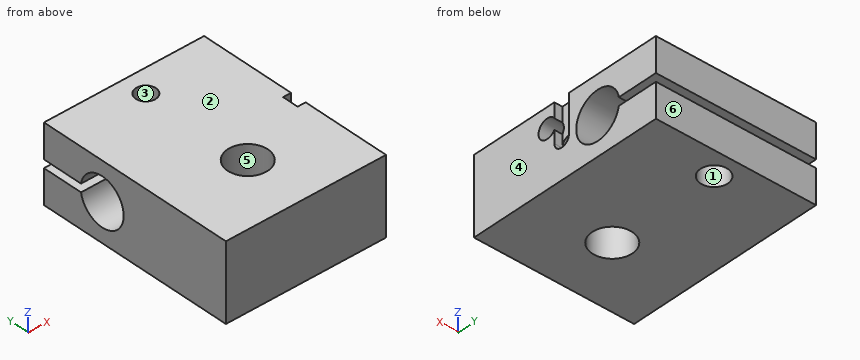
```python
from build123d import *

# Parameters (mm, degrees)
F0_W     = 20
F0_H     = 25
F0_R     = 2.5
F0_R_2   = 1.25
F1_DEPTH = 4.75
F3_DEPTH = 20.001
F4_R     = 1.7
F5_DEPTH = 4.25
F6_R     = 1
F6_R_2   = 1.190625
F7_DEPTH = 7
F8_W     = 2
F8_H     = 4.7499998814
F9_DEPTH = 1


with BuildPart() as f1:
    # F0 (on Top) → F1 (new body, symmetric)
    with BuildSketch(Plane.XY):
        Rectangle(F0_W, F0_H)
        with Locations((0, -4.5)):
            Circle(F0_R, mode=Mode.SUBTRACT)
        with Locations((0, 9.5)):
            Circle(F0_R_2, mode=Mode.SUBTRACT)
    extrude(amount=F1_DEPTH, both=True)

    # F2 (on face) → F3 (cut, through all)
    with BuildSketch(Plane.YZ.offset(10)):
        with BuildLine():
            ThreePointArc((7.407318352, -0.5), (7.43931022, -0.2509092082), (7.45, 0))
            ThreePointArc((7.45, 0), (7.43931022, 0.2509092082), (7.407318352, 0.5))
            Line((7.407318352, 0.5), (7.407318352, -0.5))
        make_face()
        with BuildLine():
            ThreePointArc((7.407318352, 0.5), (7.43931022, 0.2509092082), (7.45, 0))
            ThreePointArc((7.45, 0), (7.43931022, -0.2509092082), (7.407318352, -0.5))
            Line((7.407318352, -0.5), (12.5, -0.5))
            Line((12.5, -0.5), (12.5, 0.5))
            Line((12.5, 0.5), (7.407318352, 0.5))
        make_face()
        with BuildLine():
            Line((7.407318352, -0.5), (7.407318352, 0.5))
            ThreePointArc((7.407318352, 0.5), (1.55, 0), (7.407318352, -0.5))
        make_face()
    extrude(amount=-F3_DEPTH, mode=Mode.SUBTRACT)

    # F4 (on face) → F5 (cut, through all)
    with BuildSketch(Plane(origin=(0, 0, -4.75), x_dir=(1, 0, 0), z_dir=(0, 0, -1))):
        with Locations((0, -9.5)):
            Circle(F4_R)
    extrude(amount=-F5_DEPTH, mode=Mode.SUBTRACT)

    # F6 (on face) → F7 (cut)
    with BuildSketch(Plane.YZ.offset(10)):
        with Locations((-0.45, 0)):
            Circle(F6_R)
        with Locations((-2.4343134833, 2.25)):
            Circle(F6_R_2)
    extrude(amount=-F7_DEPTH, mode=Mode.SUBTRACT)

    # F8 (on face) → F9 (cut)
    with BuildSketch(Plane.YZ.offset(10)):
        with Locations((-0.45, 2.3750000593)):
            Rectangle(F8_W, F8_H)
    extrude(amount=-F9_DEPTH, mode=Mode.SUBTRACT)


solid = f1.part
```
Check sheet for the modelled part. Datum: model origin and axes. Units: mm. Face numbers are marked on the shaded views. A direction names the side the tool comes from. Give positions to 0.01 mm unless a question says otherwise; leave off trailing zeros. Write each loop counter-clockwise with the first axis right and the second up, starting at its lowest first coordinate (ties: lowest second). Pieces come first, ordered by that corner, then holes.
Item 1: Cross-section at B-B (x = 0). Enter the section's corners in (y, z), and give its area (3 significant figures).
Item 2: Scan lines: L1, parallel to Y at x = 0, z = 3; L2, parallel to X at y = 9.5, z = -1.95; L3, parallel to Y at x = 0.25, z = 1. Record each from-to range of solid material in increasing order.
Item 3: Cross-section at C-C (y = 9.5). Enter the section's corners in (x, z), and give its area (3 significant figures).
Item 4: Cross-section at A-A (y = 4.5). Enter the section's corners in (x, z), and give its area (3 significant figures).
Item 5: Draft check along Y on the marked faces 3, 4, 5 and 6. Enter one of: released by +Y, released by -Y, zero draft, split by the parting line, or undercut.
Item 6: Cross-section at D-D (z = 2.25). Enter the section's corners in (x, y), and give its area (3 significant figures).
Item 7: Access from +Z, -Z, +X, -X, +Y, -Y to the whole of each face (thin tool, end or side, straight path). Record for the marked faces 1 and 2.
Report:
1. outline: (-12.5, -4.75) - (-7, -4.75) - (-7, 4.75) - (-12.5, 4.75) - close; (-2, -4.75) - (7.8, -4.75) - (7.8, -0.5) - (7.41, -0.5) arc R2.95 cw (long way) to (7.41, 0.5) - (8.25, 0.5) - (8.25, 4.75) - (-2, 4.75) - close; (10.75, 0.5) - (12.5, 0.5) - (12.5, 4.75) - (10.75, 4.75) - close; (11.2, -4.75) - (12.5, -4.75) - (12.5, -0.5) - (11.2, -0.5) - close
1. area: 133 mm2
2. L1: y = -12.5 to -7, -2 to 8.25, 10.75 to 12.5
2. L2: x = -10 to -1.7, 1.7 to 10
2. L3: y = -12.5 to -6.99, -2.01 to 1.72, 7.28 to 8.28, 10.72 to 12.5
3. outline: (-10, -4.75) - (-1.7, -4.75) - (-1.7, -0.5) - (-10, -0.5) - close; (-10, 0.5) - (-1.25, 0.5) - (-1.25, 4.75) - (-10, 4.75) - close; (1.25, 0.5) - (10, 0.5) - (10, 4.75) - (1.25, 4.75) - close; (1.7, -4.75) - (10, -4.75) - (10, -0.5) - (1.7, -0.5) - close
3. area: 145 mm2
4. outline: (-10, -4.75) - (10, -4.75) - (10, -2.95) - (-10, -2.95) - close; (-10, 2.95) - (10, 2.95) - (10, 4.75) - (-10, 4.75) - close
4. area: 72.0 mm2
5. face 3: undercut
5. face 4: zero draft
5. face 5: undercut
5. face 6: released by +Y
6. outline: (-10, -12.5) - (10, -12.5) - (10, -3.62) - (3, -3.62) - (3, -1.24) - (9, -1.24) - (9, 0.55) - (10, 0.55) - (10, 2.59) - (-10, 2.59) - close; (-10, 6.41) - (10, 6.41) - (10, 12.5) - (-10, 12.5) - close; hole circle Ø5 at (0, -4.5); hole circle Ø2.5 at (0, 9.5)
6. area: 381 mm2
7. face 1: -Z
7. face 2: +Z, +X, -X, +Y, -Y
